Design review of the part shown in the three views and the two pictorial views. Dimensions are in mm from the part's minimum x, y and z. Round coordinates to 2 decimals unless told otherwise and drop trailing zeros. Order: outer loops, then holes, each group sorted by start corner. A loop starts at its lowest first (then second) coordinate and runs counter-clockwise, first axis right, second up. Notation, with made-up numbers: M 53.25,29.5 L 63.25,29.5 A15 cw 63.25,46.5 Z; hole C -34.75,-5 d9. An arc over 180 degrees is marked long. Use a Markdown table: item, result. Add a question column.
(1) Take a section at D-D (z = 26). Write out the cut boundary in (x, y).
(2) Take a section at C-C (z = 50.5). Write out the cut boundary in (x, y).
(3) For pin 1 (1 mm diameter, centred on y = 18, z = 53, fed in from +X); pin 2 (1.5 mm diameter, centred on x = 32, z = 14, fed in from +Y); pin 3 (0.6 mm diameter, centred on y = 26.5, z = 0.5, fed in from +X); pin 4 (6 mm diameter, centred on x = 9.5, y = 26, fed in from -Z), all flat-tipped, find the tip position at first contact; note any pin that passes through.
(4) Take a section at B-B (x = 7). Write out the cut boundary in (y, z), then the cut area to 3 significant figures.
(5) The part is to be moulded in two halves that separate along X. For the marked faces 1, 2 and 3, say which applies: released by +X, released by -X, zero draft, split by the parting line, or undercut.
(6) Take a section at A-A (y = 18.5). Write out the cut boundary in (x, z), then the cut area to 3 significant figures.
(7) To check wall thickness, follow probe 1 along Z at (x, y) = (33, 8); probe 2 along Z at (x, y) = (10, 27.5); probe 3 along Y at (x, z) = (30, 22.5). State the ranges of each line that lie inside material, in increasing order. Write a range as from..to.
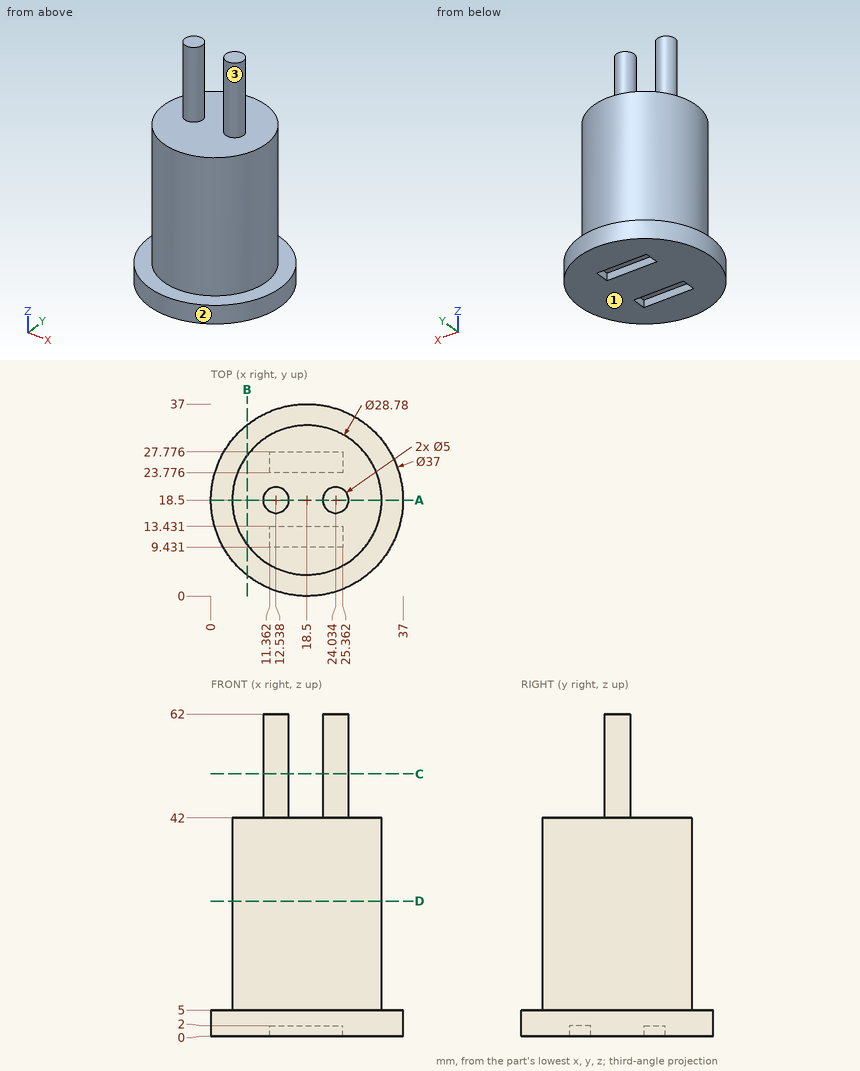
Verdict:
| question | item | result |
|---|---|---|
| 1 | outline | C 18.5,18.5 d28.78 |
| 2 | outline | C 12.54,18.5 d5; C 24.03,18.5 d5 |
| 3 | pin 1 | stops at x = 26.53 |
| 3 | pin 2 | stops at y = 25.17 |
| 3 | pin 3 | stops at x = 35.32 |
| 3 | pin 4 | stops at z = 0 |
| 4 | outline | M 4.01,0 L 32.99,0 L 32.99,5 L 27.15,5 L 27.15,42 L 9.85,42 L 9.85,5 L 4.01,5 Z |
| 4 | area | 785 mm^2 |
| 5 | face 1 | zero draft |
| 5 | face 2 | split by the parting line |
| 5 | face 3 | undercut |
| 6 | outline | M 0,0 L 37,0 L 37,5 L 32.89,5 L 32.89,42 L 26.53,42 L 26.53,62 L 21.53,62 L 21.53,42 L 15.04,42 L 15.04,62 L 10.04,62 L 10.04,42 L 4.11,42 L 4.11,5 L 0,5 Z |
| 6 | area | 1,450 mm^2 |
| 7 | probe 1 | z = 0..5 |
| 7 | probe 2 | z = 0..42 |
| 7 | probe 3 | y = 9.85..27.15 |
